Part model, mm, in its own coordinate system. Face numbers are marked on the shaded views. A direction names the side the tool comes from. Round coordinates to 2 decimals unless told otherwise and drop trailing zeros. Loops run counter-clockwise (first coordinate to the right, second up) from the corner with the lowest first, then second, coordinate; pieces in that order, holes last. Notation, with made-up numbers: (-12.75, -8) - (18.25, -8) arc R19 ccw to (18.25, 29) - close; hole circle Ø7 at (3, 81.5). An arc over 180 degrees is marked (long way). Put each result on its own line as item: value.
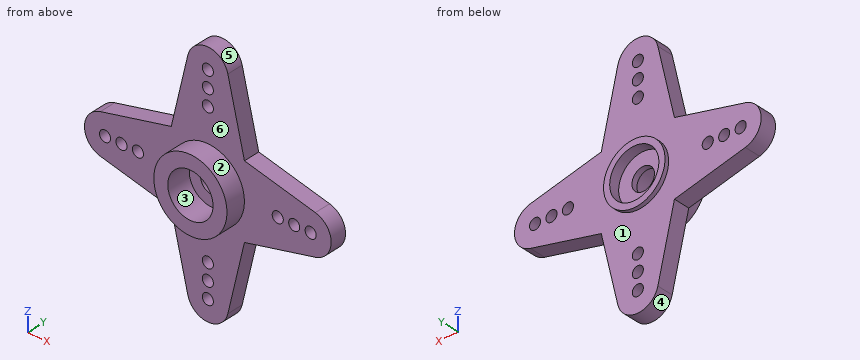
Autodesk Inventor part; units mm, degrees
ref_plane "YZ Plane" through (0, 0, 0) normal (1, 0, 0) x (0, 1, 0)
ref_plane "XZ Plane" through (0, 0, 0) normal (0, 1, 0) x (-1, 0, 0)
ref_plane "XY Plane" through (0, 0, 0) normal (0, 0, 1) x (1, 0, 0)
sketch "Sketch1" plane through (0, 0, 0) normal (0, 1, 0) x (-1, 0, 0)
  circle A0 centre (0, 0) radius 4.45
  circle A1 centre (12.5, 0) radius 2.5
  circle A2 centre (0, -12.5) radius 2.5
  line L0 (4.45, -4.45) -> (13.0693, -2.4343)
  line L1 (4.45, -4.45) -> (2.4343, -13.0693)
  circle A3 centre (12.5, 0) radius 2.5
  circle A4 centre (0, 12.5) radius 2.5
  line L2 (4.45, 4.45) -> (13.0693, 2.4343)
  line L3 (4.45, 4.45) -> (2.4343, 13.0693)
  circle A5 centre (-12.5, 0) radius 2.5
  line L4 (-4.45, -4.45) -> (-13.0693, -2.4343)
  line L5 (-4.45, -4.45) -> (-2.4343, -13.0693)
  line L6 (-4.45, 4.45) -> (-13.0693, 2.4343)
  line L7 (-4.45, 4.45) -> (-2.4343, 13.0693)
  dimension "d2" = 5
  dimension "d0" = 8.9
extrude "Extrusion1" add sketch "Sketch1" along normal blind 2 contours A0 | A1 | A1 L0 L1 A2 L5 L4 A5 L6 L7 A4 L3 L2 | A4 | A2 | A5
sketch "Sketch2" plane through (0, 2, 0) normal (0, 1, 0) x (1, 0, 0)
  circle A0 centre (0, 0) radius 3.74
  dimension "d8" = 7.48
extrude "Extrusion2" add sketch "Sketch2" along normal blind 0.5
sketch "Sketch3" plane through (0, 2.5, 0) normal (0, 1, 0) x (1, 0, 0)
  circle A0 centre (0, 0) radius 2.99
  dimension "d11" = 5.98
extrude "Extrusion3" cut sketch "Sketch3" against normal blind 1.25
sketch "Sketch4" plane through (0, 1.25, 0) normal (0, 1, 0) x (1, 0, 0)
  circle A0 centre (0, 0) radius 1.37
  dimension "d14" = 2.74
extrude "Extrusion4" cut sketch "Sketch4" against normal blind 0.69
sketch "Sketch5" plane through (0, 0, 0) normal (0, -1, 0) x (1, 0, 0)
  circle A0 centre (0, 0) radius 4.45
  dimension "d17" = 8.9
extrude "Extrusion5" add sketch "Sketch5" along normal blind 2.44
sketch "Sketch6" plane through (0, -2.44, 0) normal (0, -1, 0) x (1, 0, 0)
  circle A0 centre (0, 0) radius 2.75
  dimension "d20" = 5.5
extrude "Extrusion6" cut sketch "Sketch6" against normal blind 3
sketch "Sketch7" plane through (0, 2, 0) normal (0, 1, 0) x (1, 0, 0)
  circle A0 centre (0, 8.5) radius 0.675
  circle A1 centre (0, 10.5) radius 0.675
  arc A2 (2.4343, 13.0693) -> (-2.4343, 13.0693) centre (0, 12.5) ccw
  circle A3 centre (0, 12.5) radius 0.675
  arc A4 (-13.0693, 2.4343) -> (-13.0693, -2.4343) centre (-12.5, 0) ccw
  arc A5 (13.0693, -2.4343) -> (13.0693, 2.4343) centre (12.5, 0) ccw
  circle A6 centre (0, -8.5) radius 0.675
  circle A7 centre (0, -10.5) radius 0.675
  circle A8 centre (0, -12.5) radius 0.675
  circle A9 centre (0, 0) radius 3.74
  circle A10 centre (8.5, 0) radius 0.675
  circle A11 centre (0, 0) radius 1.37
  circle A12 centre (10.5, 0) radius 0.675
  circle A13 centre (12.5, 0) radius 0.675
  arc A14 (-2.4343, -13.0693) -> (2.4343, -13.0693) centre (0, -12.5) ccw
  circle A15 centre (-8.5, 0) radius 0.675
  circle A16 centre (-10.5, 0) radius 0.675
  circle A17 centre (-12.5, 0) radius 0.675
  dimension "d24" = 1.35
  dimension "d26" = 1.35
  dimension "d28" = 1.35
  dimension "d30" = 1.35
  dimension "d32" = 1.35
  dimension "d34" = 1.35
extrude "Extrusion7" cut sketch "Sketch7" against normal blind 2 contours A0 | A1 | A3 | A6 | A7 | A8 | A10 | A12 | A13 | A15 | A16 | A17
properties part number "MMAE 232 Assignment 2_Servo Horn 5 - Dylan Tamras"
1. Band-saw the part on B-B (z = 8.5). List the corners of the cut face in (x, y) (3 decimals), plus the area to 3 significant figures.
A:
outline: (-3.503, 0) - (-0.675, 0) - (-0.675, 2) - (-3.503, 2) - close; (0.675, 0) - (3.503, 0) - (3.503, 2) - (0.675, 2) - close
area: 11.3 mm²
2. Band-saw the part on A-A (x = -12.5). List the corners of the cut face in (y, z) (3 decimals), plus the area to 3 significant figures.
A:
outline: (0, -2.567) - (2, -2.567) - (2, -0.675) - (0, -0.675) - close; (0, 0.675) - (2, 0.675) - (2, 2.567) - (0, 2.567) - close
area: 7.57 mm²
3. Band-saw the part on D-D (x = 1.75). List the corners of the cut face in (y, z), plus the area to 3 significant figures.
A:
outline: (-2.44, -4.09) - (0, -4.09) - (0, -14.29) - (2, -14.29) - (2, -3.31) - (2.5, -3.31) - (2.5, -2.42) - (1.25, -2.42) - (1.25, 2.42) - (2.5, 2.42) - (2.5, 3.31) - (2, 3.31) - (2, 14.29) - (0, 14.29) - (0, 4.09) - (-2.44, 4.09) - (-2.44, 2.12) - (0.56, 2.12) - (0.56, -2.12) - (-2.44, -2.12) - close
area: 61.6 mm²
4. Two-plate mould, pull along Z, no slides. Class the marked faces 1, 2, 3 and 4: pulls with the +Z half, pulls with the -Z half, needs draft (parallel to the pull), parting line crosses it, or undercut.
A:
face 1: needs draft
face 2: parting line crosses it
face 3: undercut
face 4: pulls with the -Z half
5. Tool access for the marked faces 5 and 6: list every direction of +Z, -Z, +X, -X, +Y, -Y with a clear straight run to the whole face (end or side of a thin tool).
A:
face 5: +Z, +Y, -Y
face 6: -Y
6. Probe line 1 along X through (y, z) = (0.6, 12.5) (3 decimals); line 2 along Z through (x, y) = (1.75, 0.45); line 3 along Y through (x, z) = (2, 7.25). List the from-to ranges inside material, lowest first. Write a range as [from, to].
A:
line 1: x = [-2.567, -0.675], [0.675, 2.567]
line 2: z = [-14.29, -2.12], [2.12, 14.29]
line 3: y = [0, 2]
7. Band-saw the part on C-C (y = -0.4). List the corners of the cut face in (x, z).
A:
outline: circle Ø8.9 at (0, 0); hole circle Ø5.5 at (0, 0)
8. Pin check, flat tips, straight feed: P1, Ø5, axis at x = 9, z = 7, coming from the -Y side; P2, Ø1.6, axis at x = -10.5, z = 0, coming from the -Y side; P3, Ø2, axis at x = 7, y = 0.5, coming from the +Z side; P4, Ø5, axis at x = 0, z = 0, coming from the -Y side. Stop position of each tip, or through.
A:
P1: passes through
P2: stops at y = 0
P3: stops at z = 4.09
P4: stops at y = 0.56
